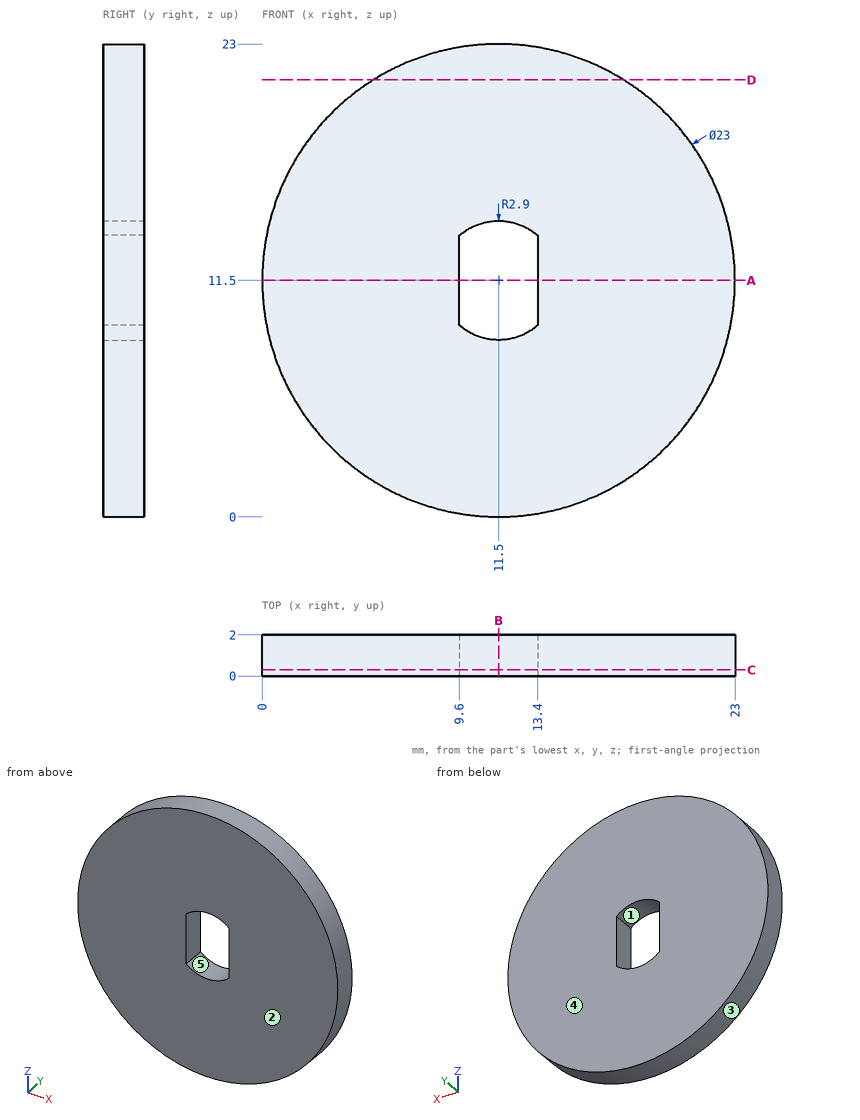
Print and shaded views of the part. All mm, measured from the part's lowest x, y and z. A direction names the side the tool comes from. Give positions to 0.01 mm unless a question says otherwise; leave off trailing zeros. Order: outer loops, then holes, each group sorted by start corner. A loop starts at its lowest first (then second) coordinate and runs counter-clockwise, first axis right, second up. Notation, with made-up numbers: (-12.75, 49) - (42.25, 49) arc R14 ccw to (42.25, 63) - close; hole circle Ø6 at (27, -15). An arc over 180 degrees is marked (long way). One line per item, written item: value.
Item 1: Tool access for the marked faces 1 and 2: list every direction of +Z, -Z, +X, -X, +Y, -Y with a clear straight run to the whole face (end or side of a thin tool).
Response values:
face 1: +Y, -Y
face 2: +Z, -Z, +X, -X, -Y
Item 2: Pin check, flat tip, straight feed: pin 1 Ø1 at (y, z) = (0.5, 15) entering from +X. Stop position of the tip, or through.
Response values:
pin 1: x = 22.6
Item 3: Slice it at C-C (y = 0.3). List the corners of the cut face in (x, z), then the cut area to 3 significant figures.
Response values:
outline: circle Ø23 at (11.5, 11.5); hole (9.6, 9.31) arc R2.9 ccw to (13.4, 9.31) - (13.4, 13.69) arc R2.9 ccw to (9.6, 13.69) - close
area: 395 mm2
Item 4: Slice it at D-D (z = 21.25). List the corners of the cut face in (x, y).
Response values:
outline: (5.4, 0) - (17.6, 0) - (17.6, 2) - (5.4, 2) - close
Item 5: Wall check: line 1 (X direction, y = 1.4, z = 11.75); line 2 (Z direction, x = 11.75, y = 1.7); line 3 (X direction, y = 1, z = 12.75). Give the ranges that are in metal, low to high.
Response values:
line 1: 0 to 9.6, 13.4 to 23
line 2: 0 to 8.61, 14.39 to 23
line 3: 0.07 to 9.6, 13.4 to 22.93
Item 6: Slice it at A-A (z = 11.5). List the corners of the cut face in (x, y), then the cut area to 3 significant figures.
Response values:
outline: (0, 0) - (9.6, 0) - (9.6, 2) - (0, 2) - close; (13.4, 0) - (23, 0) - (23, 2) - (13.4, 2) - close
area: 38.4 mm2
Item 7: Slice it at B-B (x = 11.5). List the corners of the cut face in (y, z), then the cut area to 3 significant figures.
Response values:
outline: (0, 0) - (2, 0) - (2, 8.6) - (0, 8.6) - close; (0, 14.4) - (2, 14.4) - (2, 23) - (0, 23) - close
area: 34.4 mm2
Item 8: Two-plate mould, pull along X, no slides. Class the marked faces 3, 4 and 5: released by +X, released by -X, zero draft, split by the parting line, or undercut.
Response values:
face 3: split by the parting line
face 4: zero draft
face 5: undercut
